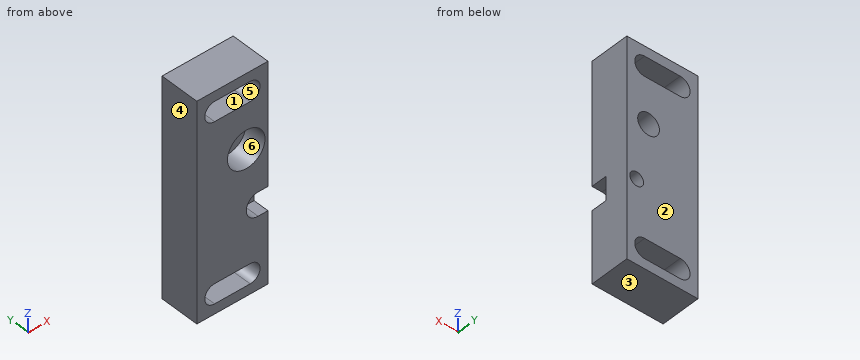
```python
from build123d import *

# Parameters (mm, degrees)
SKETCH1_W           = 18
SKETCH1_H           = 55
BOSS_EXTRUDE1_DEPTH = 10
SKETCH2_R           = 2.75
SKETCH2_R_2         = 1.75
CUT_EXTRUDE1_DEPTH  = 31.61453903
SKETCH3_R           = 4.75
CUT_EXTRUDE2_DEPTH  = 5.5
CUT_EXTRUDE3_START  = -4
SKETCH4_R           = 1.75
CUT_EXTRUDE3_DEPTH  = 4
SKETCH5_R           = 2.5
CUT_EXTRUDE4_DEPTH  = 31.61453903


with BuildPart() as part:
    # Sketch1 → Boss-Extrude1 (new body)
    with BuildSketch(Plane(origin=(0, 0, 0), x_dir=(1, 0, 0), z_dir=(0, 1, 0))):
        Rectangle(SKETCH1_W, SKETCH1_H)
    extrude(amount=BOSS_EXTRUDE1_DEPTH)

    # Sketch2 → Cut-Extrude1 (cut, through all)
    with BuildSketch(Plane(origin=(0, 10, 0), x_dir=(1, 0, 0), z_dir=(0, 1, 0))):
        with Locations(Location((3.5, -8.75, 0), (0, 0, 270))):
            Circle(SKETCH2_R)
        with Locations(Location((6.5, 6.4, 0), (0, 0, 270))):
            Circle(SKETCH2_R_2)
    extrude(amount=-CUT_EXTRUDE1_DEPTH, mode=Mode.SUBTRACT)

    # Sketch3 → Cut-Extrude2 (cut)
    with BuildSketch(Plane.XZ):
        with Locations(Location((3.5, 8.75, 0), (0, 0, 270))):
            Circle(SKETCH3_R)
    extrude(amount=-CUT_EXTRUDE2_DEPTH, mode=Mode.SUBTRACT)

    # Sketch4 → Cut-Extrude3 (cut)
    # profile 1 of 3: a face of its own
    with BuildSketch(Plane.XZ.offset(CUT_EXTRUDE3_START)):
        with BuildLine():
            ThreePointArc((6.5, -3.4), (3.5, -6.4), (6.5, -9.4))
            ThreePointArc((6.5, -9.4), (7.918637165, -9.043382037), (9, -8.058312395))
            Line((9, -8.058312395), (9, -4.741687605))
            ThreePointArc((9, -4.741687605), (7.918637165, -3.756617963), (6.5, -3.4))
        make_face()
        with Locations(Location((6.5, -6.4, 0), (0, 0, 90))):
            Circle(SKETCH4_R, mode=Mode.SUBTRACT)
    # profile 2 of 3: a face of its own
    with BuildSketch(Plane.XZ.offset(CUT_EXTRUDE3_START)):
        with BuildLine():
            ThreePointArc((9, -8.058312395), (7.918637165, -9.043382037), (6.5, -9.4))
            Line((6.5, -9.4), (9, -9.4))
            Line((9, -9.4), (9, -8.058312395))
        make_face()
    # profile 3 of 3: a face of its own
    with BuildSketch(Plane.XZ.offset(CUT_EXTRUDE3_START)):
        with BuildLine():
            Line((9, -3.4), (6.5, -3.4))
            ThreePointArc((6.5, -3.4), (7.918637165, -3.756617963), (9, -4.741687605))
            Line((9, -4.741687605), (9, -3.4))
        make_face()
    extrude(amount=CUT_EXTRUDE3_DEPTH, mode=Mode.SUBTRACT)

    # Sketch5 → Cut-Extrude4 (cut, through all)
    with BuildSketch(Plane(origin=(0, 0, 0), x_dir=(1, 0, 0), z_dir=(0, 1, 0))):
        with Locations((-4.5, 22.5)):
            Circle(SKETCH5_R)
        with BuildLine():
            Line((4.5, 25), (-4.5, 25))
            ThreePointArc((-4.5, 25), (-2.732233047, 24.267766953), (-2, 22.5))
            ThreePointArc((-2, 22.5), (-2.732233047, 20.732233047), (-4.5, 20))
            Line((-4.5, 20), (4.5, 20))
            ThreePointArc((4.5, 20), (2, 22.5), (4.5, 25))
        make_face()
        with Locations((4.5, 22.5)):
            Circle(SKETCH5_R)
        with Locations((-4.5, -22.5)):
            Circle(SKETCH5_R)
        with BuildLine():
            ThreePointArc((4.5, -25), (2, -22.5), (4.5, -20))
            Line((4.5, -20), (-4.5, -20))
            ThreePointArc((-4.5, -20), (-2.732233047, -20.732233047), (-2, -22.5))
            ThreePointArc((-2, -22.5), (-2.732233047, -24.267766953), (-4.5, -25))
            Line((-4.5, -25), (4.5, -25))
        make_face()
        with Locations((4.5, -22.5)):
            Circle(SKETCH5_R)
    extrude(amount=CUT_EXTRUDE4_DEPTH, mode=Mode.SUBTRACT)


solid = part.part
```
Can you work these out from the model? Positions are in its coordinate system, mm. Face numbers are marked on the shaded views. A direction names the side the tool comes from. Give positions to 0.01 mm unless a question says otherwise; leave off trailing zeros. Loops run counter-clockwise (first coordinate to the right, second up) from the corner with the lowest first, then second, coordinate; pieces in that order, holes last. Notation, with made-up numbers: M 68,-8 L 74,-8 A8 ccw 74,-4 Z; hole C -21,2 d5. An arc over 180 degrees is marked long. Use CSV: the item, a comma, the result in double quotes. Start each with the question number.
1. Imagine slicing it at B-B, the plane x = -2.5. Write out the boundary of the cut face in (y, z).
2. On a 3-axis mill with a long thin cutter (end or side, diameter ignored), from which of +Z, -Z, +X, -X, +Y, -Y can I reach the whole of each face in a straight line? I mean the marked faces 1 and 2. Say none if no direction works.
3. If we mould it in two halves opening along X, with no side actions, what happens to the marked faces 3, 4, 5 and 6? For each: released by +X, released by -X, zero draft, split by the parting line, or undercut.
4. If I drill on L1, parallel to Z at x = -4.5, y = 7.5; L2, parallel to Z at x = 4, y = 8; L3, parallel to Z at x = 1.5, y = 4.5, over which ranges is the centre line in solid material (lowest first)?
5. Imagine slicing it at D-D, the plane x = 3. Write out the boundary of the cut face in (y, z).
6. Imagine slicing it at A-A, the plane z = -20.5. Write out the boundary of the cut face in (x, y).
7. Imagine slicing it at C-C, the plane y = 4.5. Write out the boundary of the cut face in (x, z), plus the area to 3 significant figures.
8. For P1, Ø7.5, axis at x = 2.5, z = 9, coming from the -Y side; P2, Ø4.5, axis at x = 6.5, z = -6.4, coming from the -Y side; P3, Ø5, axis at x = 3.5, z = 8.75, coming from the +Y side, each with a flat end and sliding along its axis, tell me the tip position at first contact or that it passes through.
Response values:
1,outline,"M 0,-27.5 L 10,-27.5 L 10,-25 L 0,-25 Z; M 0,-20 L 10,-20 L 10,20 L 0,20 Z; M 0,25 L 10,25 L 10,27.5 L 0,27.5 Z"
2,face 1,"+Y, -Y"
2,face 2,"+Z, -Z, +X, -X, +Y"
3,face 3,"zero draft"
3,face 4,"released by -X"
3,face 5,"undercut"
3,face 6,"undercut"
4,L1,"-27.5 to -25, -20 to 20, 25 to 27.5"
4,L2,"-27.5 to -25, -20 to 6.05, 11.45 to 20, 25 to 27.5"
4,L3,"-27.5 to -25, -20 to 4.44, 13.06 to 20, 25 to 27.5"
5,outline,"M 0,-27.5 L 10,-27.5 L 10,-25 L 0,-25 Z; M 0,-20 L 10,-20 L 10,6.05 L 5.5,6.05 L 5.5,4.03 L 0,4.03 Z; M 0,13.47 L 5.5,13.47 L 5.5,11.45 L 10,11.45 L 10,20 L 0,20 Z; M 0,25 L 10,25 L 10,27.5 L 0,27.5 Z"
6,outline,"M -9,0 L -6,0 L -6,10 L -9,10 Z; M 6,0 L 9,0 L 9,10 L 6,10 Z"
7,outline,"M -9,-27.5 L 9,-27.5 L 9,27.5 L -9,27.5 Z; hole M -4.5,-25 L 4.5,-25 A2.5 ccw 4.5,-20 L -4.5,-20 A2.5 ccw Z; hole M -4.5,20 L 4.5,20 A2.5 ccw 4.5,25 L -4.5,25 A2.5 ccw Z; hole C 3.5,8.75 d9.5; hole C 6.5,-6.4 d3.5"
7,area,"780 mm^2"
8,P1,"y = 0"
8,P2,"y = 4"
8,P3,"through"
